from build123d import *

# Parameters (mm, degrees)
BOSS_EXTRUDE1_START = 5
BOSS_EXTRUDE1_DEPTH = 57
SKETCH8_W           = 5
SKETCH8_H           = 3
REVOLVE1_ANGLE      = 90
SKETCH9_W           = 63.56376225
SKETCH9_H           = 92.375008695
SKETCH9_W_2         = 66.279802766
SKETCH9_H_2         = 103.815770587
CUT_EXTRUDE2_DEPTH  = 100
CUT_EXTRUDE3_DEPTH  = 100
CHAMFER4_SIZE       = 3
CHAMFER5_SIZE       = 3
CHAMFER7_SIZE       = 3
CHAMFER10_SIZE      = 3


with BuildPart() as part:
    # Sketch1 → Boss-Extrude1 (new body)
    with BuildSketch(Plane.XY.offset(BOSS_EXTRUDE1_START)):
        with BuildLine():
            Line((-4.330127019, -7.5), (-11.330127019, -19.624355653))
            ThreePointArc((-11.330127019, -19.624355653), (-11.829629131, -20.830260427), (-12, -22.124355653))
            Line((-12, -22.124355653), (-12, -84))
            ThreePointArc((-12, -84), (-10.535533906, -87.535533906), (-7, -89))
            Line((-7, -89), (7, -89))
            ThreePointArc((7, -89), (10.535533906, -87.535533906), (12, -84))
            Line((12, -84), (12, -22.124355653))
            ThreePointArc((12, -22.124355653), (11.829629131, -20.830260427), (11.330127019, -19.624355653))
            Line((11.330127019, -19.624355653), (4.330127019, -7.5))
            ThreePointArc((4.330127019, -7.5), (0, -5), (-4.330127019, -7.5))
        make_face()
    extrude(amount=BOSS_EXTRUDE1_DEPTH)

    # Sketch7 → Cut-Revolve2 (revolve, cut)
    with BuildSketch(Plane(origin=(0, 0, 0), x_dir=(0, 0, -1), z_dir=(1, 0, 0))):
        Polygon((-73.391777599, -41), (-62, -41), (-46, -41), (-46, -65), (-30, -65), (-30, -89), (-30, -99.200268773), (-73.391777599, -99.200268773), align=None)
        Polygon((-28.5, -77), (-30, -75.5), (-30, -78.5), align=None)
        Polygon((-38, -63.5), (-36.5, -65), (-39.5, -65), align=None)
        Polygon((-44.5, -53), (-46, -54.5), (-46, -51.5), align=None)
        Polygon((-54, -39.5), (-52.5, -41), (-55.5, -41), align=None)
    revolve(axis=Axis((0, 0, 0), (0, 0, 1)), mode=Mode.SUBTRACT)

    # Sketch8 → Revolve1 (revolve, symmetric)
    with BuildSketch(Plane(origin=(0, 0, 0), x_dir=(0, 0, -1), z_dir=(1, 0, 0))) as revolve1_sk:
        with Locations((-2.5, -35.5)):
            Rectangle(SKETCH8_W, SKETCH8_H)
        with Locations((-2.5, -27.5)):
            Rectangle(SKETCH8_W, SKETCH8_H)
        with Locations((-2.5, -43.5)):
            Rectangle(SKETCH8_W, SKETCH8_H)
        with Locations((-2.5, -51.5)):
            Rectangle(SKETCH8_W, SKETCH8_H)
        with Locations((-2.5, -59.5)):
            Rectangle(SKETCH8_W, SKETCH8_H)
        with Locations((-2.5, -67.5)):
            Rectangle(SKETCH8_W, SKETCH8_H)
        with Locations((-2.5, -75.5)):
            Rectangle(SKETCH8_W, SKETCH8_H)
    revolve(axis=Axis((0, 0, 22.869751467), (0, 0, -1)), revolution_arc=REVOLVE1_ANGLE / 2)
    revolve(revolve1_sk.sketch, axis=Axis((0, 0, 22.869751467), (0, 0, 1)), revolution_arc=REVOLVE1_ANGLE / 2)

    # Sketch9 → Cut-Extrude2 (cut)
    with BuildSketch(Plane(origin=(0, 0, 0), x_dir=(1, 0, 0), z_dir=(0, 1, 0))):
        with Locations((-43.781881125, -28.783671007)):
            Rectangle(SKETCH9_W, SKETCH9_H)
        with Locations((45.139901383, -26.868725236)):
            Rectangle(SKETCH9_W_2, SKETCH9_H_2)
    extrude(amount=-CUT_EXTRUDE2_DEPTH, mode=Mode.SUBTRACT)

    # Sketch10 → Cut-Extrude3 (cut)
    with BuildSketch(Plane(origin=(0, 0, 0), x_dir=(1, 0, 0), z_dir=(0, 1, 0))):
        with BuildLine():
            Line((12, -21), (12, -20.164136905))
            Line((12, -20.164136905), (12, -13))
            Line((12, -13), (12, -12.164136905))
            Line((12, -12.164136905), (8.601411599, -11.092566099))
            ThreePointArc((8.601411599, -11.092566099), (6.817380703, -11.387110791), (6, -13))
            Line((6, -13), (6, -20.164136905))
            ThreePointArc((6, -20.164136905), (6.817380703, -21.777026114), (8.601411599, -22.071570807))
            Line((8.601411599, -22.071570807), (12, -21))
        make_face()
        with BuildLine():
            Line((-12, -12.164136905), (-12, -13))
            Line((-12, -13), (-12, -20.164136905))
            Line((-12, -20.164136905), (-12, -21))
            Line((-12, -21), (-8.601411599, -22.071570807))
            ThreePointArc((-8.601411599, -22.071570807), (-6.817380703, -21.777026114), (-6, -20.164136905))
            Line((-6, -20.164136905), (-6, -13))
            ThreePointArc((-6, -13), (-6.817380703, -11.387110791), (-8.601411599, -11.092566099))
            Line((-8.601411599, -11.092566099), (-12, -12.164136905))
        make_face()
    extrude(amount=-CUT_EXTRUDE3_DEPTH, mode=Mode.SUBTRACT)

    # Chamfer4
    chamfer4_edges = [part.edges().sort_by_distance(p)[0] for p in [
        (12, -44.643511809, 46),
    ]]
    chamfer(chamfer4_edges, length=CHAMFER4_SIZE)

    # Chamfer5
    chamfer5_edges = [part.edges().sort_by_distance(p)[0] for p in [
        (11.829629131, -20.830260427, 62),
        (7.830127019, -13.562177826, 62),
        (0, -5, 62),
        (12, -30.66447361, 62),
        (-7.830127019, -13.562177826, 62),
        (-11.829629131, -20.830260427, 62),
        (-12, -30.66447361, 62),
    ]]
    chamfer(chamfer5_edges, length=CHAMFER5_SIZE)

    # Chamfer7
    chamfer7_edges = [part.edges().sort_by_distance(p)[0] for p in [
        (-12, -44.643511809, 46),
    ]]
    chamfer(chamfer7_edges, length=CHAMFER7_SIZE)

    # Chamfer10
    # the kernel refuses this chamfer: 3 mm, written as the material it takes off along each edge
    with BuildSketch(Plane(origin=(-12, -82.255306543, 30), x_dir=(0.9996219169112968, 0, 0.02749587661058678), z_dir=(0, 1, 0))) as chamfer10_piece_1_section:
        Polygon((CHAMFER10_SIZE * 0.999621916911, CHAMFER10_SIZE * 0.0274958766106), (-CHAMFER10_SIZE * 0.0274958766106, CHAMFER10_SIZE * 0.999621916911), (0, 0), align=None)
    chamfer10_piece_1 = extrude(amount=26.087650492, mode=Mode.PRIVATE)
    chamfer10_piece_1 = chamfer10_piece_1 - Plane(origin=(0, 0, 28.957588125), x_dir=(0, -1, 0), z_dir=(0, 0, -1)) * Cylinder(65, 65, mode=Mode.PRIVATE)
    add(chamfer10_piece_1, mode=Mode.SUBTRACT)
    with BuildSketch(Plane(origin=(-12, -91.715048964, 30), x_dir=(0.9996219169112968, 0, 0.02749587661058678), z_dir=(0, 1, 0)), Plane(origin=(12, -69.86233176, 30), x_dir=(-0.9996219169112968, 0, 0.02749587661058678), z_dir=(0, -1, 0))) as chamfer10_piece_2:
        Polygon((CHAMFER10_SIZE * 0.999621916911, CHAMFER10_SIZE * 0.0274958766106), (-CHAMFER10_SIZE * 0.0274958766106, CHAMFER10_SIZE * 0.999621916911), (0, 0), align=None)
    extrude(amount=21.852717204, mode=Mode.SUBTRACT)
    with BuildSketch(Plane(origin=(12, -56.167656051, 30), x_dir=(-0.9996219169112968, 0, 0.02749587661058678), z_dir=(0, -1, 0))) as chamfer10_piece_3_section:
        Polygon((CHAMFER10_SIZE * 0.999621916911, CHAMFER10_SIZE * 0.0274958766106), (-CHAMFER10_SIZE * 0.0274958766106, CHAMFER10_SIZE * 0.999621916911), (0, 0), align=None)
    chamfer10_piece_3 = extrude(amount=26.087650492, mode=Mode.PRIVATE)
    chamfer10_piece_3 = chamfer10_piece_3 - Plane(origin=(0, 0, 28.982814192), x_dir=(0, -1, 0), z_dir=(0, 0, -1)) * Cylinder(65, 65, mode=Mode.PRIVATE)
    add(chamfer10_piece_3, mode=Mode.SUBTRACT)


solid = part.part
Could you check a few things on this model? Use its own coordinates, in mm. A direction names the side the tool comes from. Give positions to 0.01 mm unless a question says otherwise; leave off trailing zeros. Order: outer loops, then holes, each group sorted by start corner. A loop starts at its lowest first (then second) coordinate and runs counter-clockwise, first axis right, second up.
1. Suppose I cut it at A-A (y = -70). List the corners of the cut face in (x, z) for me.
2. Will these pins go through, and if not, where does the flat tip stop? P1, Ø5.5, axis at x = 3, y = -82.5, coming from the +Z side; P2, Ø1, axis at x = -5.5, y = -24.5, coming from the -Z side; P3, Ø3.5, axis at x = -2, y = -46.5, coming from the +Z side.
3. For faces 5 (the flat face through (0, -59, 46)), 6 (the flat face through (-11, -76, 28)), 7 (the cylindrical face through (0, -65, 43)), 8 (the cylindrical face through (0, -69, 2)), which set-ups out of +Z, -Z, +X, -X, +Y, -Y let a thin tool reach every point of the face, with its end or its side?
4. I need wall thicknesses on L1, parallel to Z at x = 8, y = -60; L2, parallel to Z at x = -7.5, y = -42; L3, parallel to X at y = -63, z = 13. Which ranges of each line are inside material? Lowest first, please.
5. We'd pull the mould along Z, two halves only. Please class faces 1 (the flat face through (0, -51, 0)), 2 (the flat face through (10.277, -51.3, 21.543)), 3 (the flat face through (-6.464, -14.238, 60.521)), 4 (the cylindrical face through (0, -5, 32)): pulls with the +Z half, pulls with the -Z half, needs draft (parallel to the pull), parting line crosses it, or undercut.
6. Suppose I cut it at C-C (y = -11.5). List the corners of the cut face in (x, z) for me.
7. Suppose I cut it at B-B (z = 56.5). List the corners of the cut face in (x, y) for me.
Solved:
1. outline: (-12, 5) - (12, 5) - (12, 12.16) - (8.6, 11.09) arc R2 cw to (6, 13) - (6, 20.16) arc R2 cw to (8.6, 22.07) - (12, 21) - (12, 27) - (9, 30) - (-9, 30) - (-12, 27) - (-12, 21) - (-8.6, 22.07) arc R2 cw to (-6, 20.16) - (-6, 13) arc R2 cw to (-8.6, 11.09) - (-12, 12.16) - close
2. P1: stops at z = 30
2. P2: stops at z = 5
2. P3: stops at z = 46
3. face 5: +Z, +X, -X, -Y
3. face 6: +Z, -X, -Y
3. face 7: +Z, -Y
3. face 8: -Z
4. L1: z = 0 to 11, 22.16 to 46
4. L2: z = 0 to 11.06, 22.1 to 46
4. L3: x = -6 to 6
5. face 1: pulls with the -Z half
5. face 2: undercut
5. face 3: pulls with the +Z half
5. face 4: needs draft
6. outline: (-6.64, 5) - (6.64, 5) - (6.64, 11.53) arc R2 cw to (6, 13) - (6, 20.16) arc R2 cw to (6.64, 21.63) - (6.64, 59) - (3.18, 62) - (-3.18, 62) - (-6.64, 59) - (-6.64, 21.63) arc R2 cw to (-6, 20.16) - (-6, 13) arc R2 cw to (-6.64, 11.53) - close
7. outline: (-12, -39.2) arc R41 ccw to (12, -39.2) - (12, -22.12) arc R5 ccw to (11.33, -19.62) - (4.33, -7.5) arc R5 ccw to (-4.33, -7.5) - (-11.33, -19.62) arc R5 ccw to (-12, -22.12) - close
